from build123d import *

# Parameters (mm, degrees)
F2_C1_SIZE2 = 0.5
F2_C1_SIZE  = 0.7
F2_C2_SIZE2 = 0.7
F2_C2_SIZE  = 0.5
F2_C3_SIZE2 = 0.7
F2_C3_SIZE  = 0.5


with BuildPart() as f1:
    # F0 (on Front) → F1 (revolve)
    with BuildSketch(Plane.XZ):
        Polygon((0.7, 6), (0.7, 0), (2.9, 0), (2.9, 5.4), (3.65, 5.4), (3.65, 5), (5, 5), (5, 11.1), (1.7, 11.1), (1.7, 6), align=None)
    revolve(axis=Axis((0, 0, 5.55), (0, 0, -1)))

    # F2: chamfer of 0.7 x 0.5 on 3 edges, made by hand

    # F2_c1
    f2_c1_edges = [f1.edges().sort_by_distance(p)[0] for p in [
        (-1.7, 0, 11.1),
    ]]
    f2_c1_side = f1.faces().sort_by_distance((-1.7, 0, 11.09))[0]
    chamfer(f2_c1_edges, length=F2_C1_SIZE, length2=F2_C1_SIZE2, reference=f2_c1_side)

    # F2_c2
    f2_c2_edges = [f1.edges().sort_by_distance(p)[0] for p in [
        (-2.9, 0, 0),
    ]]
    f2_c2_side = f1.faces().sort_by_distance((-2.89, 0, 0))[0]
    chamfer(f2_c2_edges, length=F2_C2_SIZE, length2=F2_C2_SIZE2, reference=f2_c2_side)

    # F2_c3
    f2_c3_edges = [f1.edges().sort_by_distance(p)[0] for p in [
        (-5, 0, 11.1),
    ]]
    f2_c3_side = f1.faces().sort_by_distance((-4.99, 0, 11.1))[0]
    chamfer(f2_c3_edges, length=F2_C3_SIZE, length2=F2_C3_SIZE2, reference=f2_c3_side)


solid = f1.part
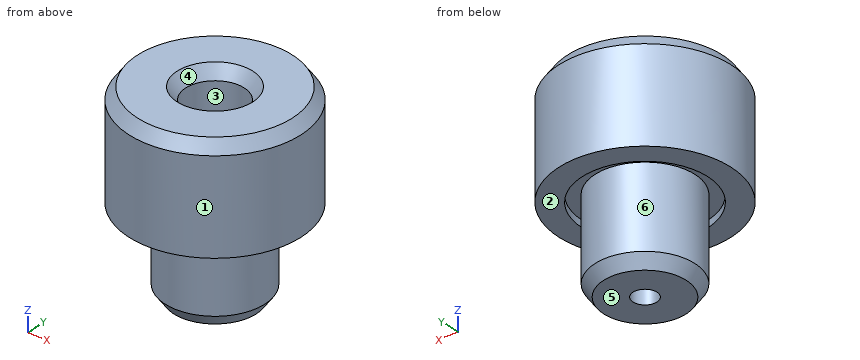
The listing builds one solid part. Answer for the finished solid, in the listing's coordinates (mm). Face numbers are marked on the shaded views. A direction names the side the tool comes from. Coordinates: 2 decimals unless noted, no trailing zeros. Write each loop counter-clockwise with the first axis right and the second up, starting at its lowest first coordinate (ties: lowest second). Pieces come first, ordered by that corner, then holes. Notation, with made-up numbers: (85.5, 59.25) - (108.5, 59.25) arc R22 ccw to (108.5, 81.25) - close; hole circle Ø2 at (4.5, -16.75). An arc over 180 degrees is marked (long way). Return JSON: item names as keys, results as strings.
1. Which of the six approach directions +Z, -Z, +X, -X, +Y, -Y give full straight-line access (tool end or side, diameter ignored) to the marked faces 5 and 6?
Final values:
{"face 5": "-Z, +X, -X, +Y, -Y", "face 6": "-Z"}
2. The part is cut by section D-D on z = 2.5. Determine the outline of the cut face in (x, y), then the cut area to 3 significant figures.
Final values:
{"outline": "circle Ø5.8 at (0, 0); hole circle Ø1.4 at (0, 0)", "area": "24.9 mm^2"}
3. The part is cut by section C-C on z = 10.75. Determine the outline of the cut face in (x, y), then the cut area to 3 significant figures.
Final values:
{"outline": "circle Ø9.5 at (0, 0); hole circle Ø3.9 at (0, 0)", "area": "58.9 mm^2"}
4. Each of these flat-tipped pins is pushed along its axis until it touches: pin 1 Ø1.5 at (y, z) = (1, 5) entering from -X; pin 2 Ø1.7 at (x, y) = (0, 0) entering from +Z; pin 3 Ø1.5 at (x, z) = (-2.5, 4) entering from +Y. Where does it stop, or does it pass through?
Final values:
{"pin 1": "x = -4.99", "pin 2": "z = 6", "pin 3": "y = 2.31"}
5. The part is cut by section A-A on y = 0. Determine the outline of the cut face in (x, z).
Final values:
{"outline": "(-5, 5) - (-3.65, 5) - (-3.65, 5.4) - (-2.9, 5.4) - (-2.9, 0.7) - (-2.4, 0) - (-0.7, 0) - (-0.7, 6) - (-1.7, 6) - (-1.7, 10.4) - (-2.2, 11.1) - (-4.5, 11.1) - (-5, 10.4) - close; (0.7, 0) - (2.4, 0) - (2.9, 0.7) - (2.9, 5.4) - (3.65, 5.4) - (3.65, 5) - (5, 5) - (5, 10.4) - (4.5, 11.1) - (2.2, 11.1) - (1.7, 10.4) - (1.7, 6) - (0.7, 6) - close"}
6. Consider line 1 along X through (y, z) = (0, 5.2); line 2 along Y through (x, z) = (0, 9.35). Determine where each line is inside the solid, lowest interval first.
Final values:
{"line 1": "-5 to -3.65, -2.9 to -0.7, 0.7 to 2.9, 3.65 to 5", "line 2": "-5 to -1.7, 1.7 to 5"}
7. For a pull along Y with two mould halves and no side action, classify the marked faces 1, 2, 3 and 4 as +Y half, -Y half, draft (parallel to the pull), parting line (faces both ways), or undercut.
Final values:
{"face 1": "parting line", "face 2": "draft", "face 3": "undercut", "face 4": "undercut"}
